The model under review builds one solid part; all positions refer to its coordinate system, in mm. A direction names the side the tool comes from. Give positions to 0.01 mm unless a question says otherwise; leave off trailing zeros. Order: outer loops, then holes, each group sorted by start corner. A loop starts at its lowest first (then second) coordinate and runs counter-clockwise, first axis right, second up.
```python
from build123d import *
from build123d.topology import SkipClean

# Parameters (mm, degrees)
SKETCH1_R               = 1.3
BOSS_EXTRUDE1_DEPTH     = 0.6
BOSS_EXTRUDE2_START     = 7.6
BOSS_EXTRUDE2_DEPTH     = 8.2
CHAMFER1_SIZE           = 0.6
CUT_EXTRUDE1_DEPTH      = 65.705177536
CUT_EXTRUDE1_DEPTH_BACK = 65.705177536
CUT_EXTRUDE2_REACH      = 66.705
SKETCH11_W              = 4.2
SKETCH11_H              = 2
FILLET1_R               = 2
CHAMFER2_SIZE           = 1.7
BOSS_EXTRUDE3_START     = 0.6
BOSS_EXTRUDE3_DEPTH     = 7
FILLET2_R               = 1


with BuildPart() as part:
    # Sketch1 → Boss-Extrude1 (new body)
    with BuildSketch(Plane(origin=(0, 0, 0), x_dir=(1, 0, 0), z_dir=(0, 1, 0))):
        with BuildLine():
            Line((-57, 0), (-56.5, 0))
            Line((-56.5, 0), (56.5, 0))
            Line((56.5, 0), (57, 0))
            ThreePointArc((57, 0), (59.121320344, 0.878679656), (60, 3))
            Line((60, 3), (60, 14))
            ThreePointArc((60, 14), (57.363961031, 20.363961031), (51, 23))
            Line((51, 23), (-51, 23))
            ThreePointArc((-51, 23), (-57.363961031, 20.363961031), (-60, 14))
            Line((-60, 14), (-60, 3))
            ThreePointArc((-60, 3), (-59.121320344, 0.878679656), (-57, 0))
        make_face()
        with Locations(Location((55, 11.43, 0), (0, 0, 270))):
            Circle(SKETCH1_R, mode=Mode.SUBTRACT)
        with Locations(Location((-55, 11.43, 0), (0, 0, 270))):
            Circle(SKETCH1_R, mode=Mode.SUBTRACT)
        with BuildLine():
            Line((-51.459505684, 21), (51.459505684, 21))
            ThreePointArc((51.459505684, 21), (55.300275809, 18.117356187), (53.605259815, 13.624242424))
            ThreePointArc((53.605259815, 13.624242424), (52.467669637, 10.840675867), (54.717391304, 8.845404804))
            ThreePointArc((54.717391304, 8.845404804), (55.989090764, 8.192398352), (56.5, 6.857254654))
            Line((56.5, 6.857254654), (56.5, 2))
            Line((56.5, 2), (49, 2))
            Line((49, 2), (49, 0.4))
            Line((49, 0.4), (-49, 0.4))
            Line((-49, 0.4), (-49, 2))
            Line((-49, 2), (-56.5, 2))
            Line((-56.5, 2), (-56.5, 6.857254654))
            ThreePointArc((-56.5, 6.857254654), (-55.989090764, 8.192398352), (-54.717391304, 8.845404804))
            ThreePointArc((-54.717391304, 8.845404804), (-52.467669637, 10.840675867), (-53.605259815, 13.624242424))
            ThreePointArc((-53.605259815, 13.624242424), (-55.300275809, 18.117356187), (-51.459505684, 21))
        make_face(mode=Mode.SUBTRACT)
    extrude(amount=BOSS_EXTRUDE1_DEPTH)

    # Sketch8 → Boss-Extrude2 (add)
    with SkipClean():  # the faces are left unmerged after this step: merging them gives an invalid solid
        with BuildSketch(Plane(origin=(0, 0, 0), x_dir=(-1, 0, 0), z_dir=(0, -1, 0)).offset(BOSS_EXTRUDE2_START)):
            with BuildLine():
                Line((-57, 0), (57, 0))
                ThreePointArc((57, 0), (59.121320344, 0.878679656), (60, 3))
                Line((60, 3), (60, 14))
                ThreePointArc((60, 14), (57.363961031, 20.363961031), (51, 23))
                Line((51, 23), (-51, 23))
                ThreePointArc((-51, 23), (-57.363961031, 20.363961031), (-60, 14))
                Line((-60, 14), (-60, 3))
                ThreePointArc((-60, 3), (-59.121320344, 0.878679656), (-57, 0))
            make_face()
            with BuildLine():
                Line((51, 22.6), (-51, 22.6))
                ThreePointArc((-51, 22.6), (-57.081118318, 20.081118318), (-59.6, 14))
                Line((-59.6, 14), (-59.6, 3))
                ThreePointArc((-59.6, 3), (-58.838477631, 1.161522369), (-57, 0.4))
                Line((-57, 0.4), (57, 0.4))
                ThreePointArc((57, 0.4), (58.838477631, 1.161522369), (59.6, 3))
                Line((59.6, 3), (59.6, 14))
                ThreePointArc((59.6, 14), (57.081118318, 20.081118318), (51, 22.6))
            make_face(mode=Mode.SUBTRACT)
        extrude(amount=-BOSS_EXTRUDE2_DEPTH)
    add(part.part.scale(1), mode=Mode.REPLACE)  # the faces are merged on a copy

    # Chamfer1
    chamfer1_edges = [part.edges().sort_by_distance(p)[0] for p in [
        (-53, 0, -0.4),
        (53, 0, -0.4),
        (-58.838477631, 0, -1.161522369),
        (-59.6, 0, -8.5),
        (-57.081118318, 0, -20.081118318),
        (0, 0, -22.6),
        (57.081118318, 0, -20.081118318),
        (59.6, 0, -8.5),
        (58.838477631, 0, -1.161522369),
    ]]
    chamfer(chamfer1_edges, length=CHAMFER1_SIZE)

    # Sketch9 → Cut-Extrude1 (cut, two sides: drawn at the far end of the back side and taken through both)
    with BuildSketch(Plane(origin=(0, 0, 0), x_dir=(0, 0, -1), z_dir=(1, 0, 0)).offset(-CUT_EXTRUDE1_DEPTH_BACK)):
        Polygon((-2, -7.6), (23, -7.6), (-2, -7.163623377), align=None)
    extrude(amount=CUT_EXTRUDE1_DEPTH + CUT_EXTRUDE1_DEPTH_BACK, mode=Mode.SUBTRACT)

    # Sketch11 → Cut-Extrude2 (cut, up to next)
    with BuildSketch(Plane.XY, mode=Mode.PRIVATE) as cut_extrude2_sk1:
        with Locations((5.35, -0.4)):
            Rectangle(SKETCH11_W, SKETCH11_H)
    cut_extrude2_tool1 = extrude(cut_extrude2_sk1.sketch, amount=-CUT_EXTRUDE2_REACH, mode=Mode.PRIVATE) & part.part
    add(cut_extrude2_tool1.solids().sort_by_distance((5.35, -0.4, 0))[0], mode=Mode.SUBTRACT)

    # Fillet1
    fillet1_edges = [part.edges().sort_by_distance(p)[0] for p in [
        (-56.5, 0.3, -2),
        (56.5, 0.3, -2),
    ]]
    fillet(fillet1_edges, radius=FILLET1_R)

    # Chamfer2
    # the kernel refuses this chamfer: 1.7 mm, written as the material it adds along each edge
    with BuildSketch(Plane(origin=(-49, -4.97186108, -0.4), x_dir=(-0.02749587661058786, 0, -0.9996219169112968), z_dir=(0, 1, 0))) as chamfer2_piece_1_section:
        Polygon((CHAMFER2_SIZE * 0.999621916911, -CHAMFER2_SIZE * 0.0274958766106), (-CHAMFER2_SIZE * 0.0274958766106, -CHAMFER2_SIZE * 0.999621916911), (0, 0), align=None)
    chamfer2_piece_1 = extrude(amount=5.57186108, mode=Mode.PRIVATE)
    chamfer2_piece_1 = split(chamfer2_piece_1, bisect_by=Plane(origin=(-48.243333333, -0.31, -0.69), z_dir=(0, 0.7071067811865475, 0.7071067811865476)), keep=Keep.TOP, mode=Mode.PRIVATE)
    add(chamfer2_piece_1)
    with BuildSketch(Plane(origin=(-49, -4.97186108, -0.4), x_dir=(-0.02749587661058786, 0, -0.9996219169112968), z_dir=(0, 1, 0))) as chamfer2_piece_2_section:
        Polygon((CHAMFER2_SIZE * 0.999621916911, -CHAMFER2_SIZE * 0.0274958766106), (-CHAMFER2_SIZE * 0.0274958766106, -CHAMFER2_SIZE * 0.999621916911), (0, 0), align=None)
    chamfer2_piece_2 = extrude(amount=5.57186108, mode=Mode.PRIVATE)
    chamfer2_piece_2 = split(chamfer2_piece_2, bisect_by=Plane(origin=(-48.705555556, 0, -1.511111111), z_dir=(0, 1, 0)), keep=Keep.TOP, mode=Mode.PRIVATE)
    chamfer2_piece_2 = split(chamfer2_piece_2, bisect_by=Plane(origin=(-48.705555556, 0.227272727, -2), z_dir=(0, 0, 1)), keep=Keep.TOP, mode=Mode.PRIVATE)
    add(chamfer2_piece_2)
    with BuildSketch(Plane(origin=(49, 0.6, -0.4), x_dir=(0.02749587661058786, 0, -0.9996219169112968), z_dir=(0, -1, 0))) as chamfer2_piece_3_section:
        Polygon((CHAMFER2_SIZE * 0.999621916911, -CHAMFER2_SIZE * 0.0274958766106), (-CHAMFER2_SIZE * 0.0274958766106, -CHAMFER2_SIZE * 0.999621916911), (0, 0), align=None)
    chamfer2_piece_3 = extrude(amount=5.57186108, mode=Mode.PRIVATE)
    chamfer2_piece_3 = split(chamfer2_piece_3, bisect_by=Plane(origin=(48.35, 0.060810811, -1.060810811), z_dir=(0, 0.7071067811865475, 0.7071067811865476)), keep=Keep.TOP, mode=Mode.PRIVATE)
    add(chamfer2_piece_3)
    with BuildSketch(Plane(origin=(49, 0.6, -0.4), x_dir=(0.02749587661058786, 0, -0.9996219169112968), z_dir=(0, -1, 0))) as chamfer2_piece_4_section:
        Polygon((CHAMFER2_SIZE * 0.999621916911, -CHAMFER2_SIZE * 0.0274958766106), (-CHAMFER2_SIZE * 0.0274958766106, -CHAMFER2_SIZE * 0.999621916911), (0, 0), align=None)
    chamfer2_piece_4 = extrude(amount=5.57186108, mode=Mode.PRIVATE)
    chamfer2_piece_4 = split(chamfer2_piece_4, bisect_by=Plane(origin=(48.705555556, 0, -1.511111111), z_dir=(0, 1, 0)), keep=Keep.TOP, mode=Mode.PRIVATE)
    chamfer2_piece_4 = split(chamfer2_piece_4, bisect_by=Plane(origin=(48.705555556, 0.227272727, -2), z_dir=(0, 0, 1)), keep=Keep.TOP, mode=Mode.PRIVATE)
    add(chamfer2_piece_4)

    # Sketch12 → Boss-Extrude3 (add)
    with BuildSketch(Plane(origin=(0, 0, 0), x_dir=(1, 0, 0), z_dir=(0, 1, 0)).offset(BOSS_EXTRUDE3_START)):
        with BuildLine():
            Line((28.272740661, 53.207055236), (36.366696717, 23))
            Line((36.366696717, 23), (35.538475773, 23))
            Line((35.538475773, 23), (27.5, 53))
            ThreePointArc((27.5, 53), (27.782842712, 53.489897949), (28.272740661, 53.207055236))
        make_face()
    extrude(amount=-BOSS_EXTRUDE3_DEPTH)

    # Fillet2
    fillet2_edges = [part.edges().sort_by_distance(p)[0] for p in [
        (36.366696717, -2.9, -23),
        (35.538475773, -2.9, -23),
    ]]
    fillet(fillet2_edges, radius=FILLET2_R)


solid = part.part
```
Item 1: Take a section at B-B (z = -11.43). Give the boundary of the cut face in (x, y).
Values found:
outline: (-60, -7.4) - (-59.6, -7.4) - (-59.6, -0.6) - (-59, 0) - (-56.3, 0) - (-56.3, 0.6) - (-60, 0.6) - close; (-53.7, 0) - (-52.4, 0) - (-52.4, 0.6) - (-53.7, 0.6) - close; (52.4, 0) - (53.7, 0) - (53.7, 0.6) - (52.4, 0.6) - close; (56.3, 0) - (59, 0) - (59.6, -0.6) - (59.6, -7.4) - (60, -7.4) - (60, 0.6) - (56.3, 0.6) - close
Item 2: For faces 1 (the cylindrical face through (55.93, 0.3, -2.6)), 2 (the flat face through (32.165, -2.851, -38.68)), 3 (the conical face through (-58.55, -0.17, -1.48)), 4 (the flat face through (60, -3, -9)), 5 (the flat face through (31.404, -2.851, -38.428)), list the 3-axis set-ups (+Z, -Z, +X, -X, +Y, -Y) from which the entire face can be reached by the end or side of a thin tool; tool diameter is ignored.
Values found:
face 1: +Y, -Y
face 2: -Z, +X, +Y, -Y
face 3: -Y
face 4: +Z, -Z, +X, +Y, -Y
face 5: -X, +Y, -Y
Item 3: Take a section at C-C (z = -31). Give the boundary of the cut face in (x, y), and give its area (3 significant figures).
Values found:
outline: (33.39, -6.4) - (34.22, -6.4) - (34.22, 0.6) - (33.39, 0.6) - close
area: 5.80 mm2
Item 4: For line 1 (X direction, y = 0.2, z = -11.43); line 2 (Z direction, x = 47.5, y = -5.25); line 3 (X direction, y = -4.5, z = -8.5), list the stretches that pass through material, from the lowest coordinate up.
Values found:
line 1: x = -60 to -56.3, -53.7 to -52.4, 52.4 to 53.7, 56.3 to 60
line 2: z = -23 to -22.6, -0.4 to 0
line 3: x = -60 to -59.6, 59.6 to 60
Item 5: Clearance check with flat-ended pins moving along their axes: pin 1 Ø4 at (x, z) = (-55, -11.43) entering from -Y; pin 2 Ø0.7 at (x, y) = (52.5, 0) entering from -Z; pin 3 Ø3 at (x, z) = (31, -40.5) entering from -Y. State where each tip first meets the part, or that it passes through.
Values found:
pin 1: stops at y = 0
pin 2: stops at z = -22.93
pin 3: stops at y = -6.4
Item 6: Draft analysis for pull direction Z (two halves, no side actions). For faces 6 (the cylindrical face through (56.29, 0.3, -11.6)), 7 (the flat face through (1, -3, 0)), 8 (the flat face through (-60, -3, -8)), state which applies: released by +Z, released by -Z, zero draft, split by the parting line, or undercut.
Values found:
face 6: undercut
face 7: released by +Z
face 8: zero draft
Item 7: Take a section at A-A (x = -29). Give the boundary of the cut face in (y, z).
Values found:
outline: (-7.6, -23) - (0.6, -23) - (0.6, -21) - (0, -21) - (0, -22) - (-0.6, -22.6) - (-7.59, -22.6) - close; (-7.21, -0.4) - (0.6, -0.4) - (0.6, 0) - (-7.2, 0) - close
